Can you work these out from the model? Positions are in its coordinate system, mm. A direction names the side the tool comes from. Give positions to 0.01 mm unless a question says otherwise; leave off trailing zeros. Write each loop counter-clockwise with the first axis right and the second up, starting at its lowest first coordinate (ties: lowest second). Pieces come first, ordered by that corner, then holes.
1. On a 3-axis mill with a long thin cutter (end or side, diameter ignored), from which of +Z, -Z, +X, -X, +Y, -Y can I reach the whole of each face in a straight line? I mean faces 1 (the flat face through (4.5, 44, 1)), 2 (the flat face through (95.5, 44, 1)), 3 (the flat face through (130, 44, 1)). Say none if no direction works.
2. Suppose I cut it at D-D (y = 62). Please give me the cut outline in (x, z).
3. If I drill on probe 1 along Y at (x, z) = (101, 1.5); probe 2 along Y at (x, z) = (25, 2.05); probe 3 along Y at (x, z) = (72, 0.75), over which ranges is the centre line in solid material (lowest first)?
4. Suppose I cut it at C-C (z = 2.4). Please give me the cut outline in (x, y).
5. Suppose I cut it at A-A (x = 25). Please give me the cut outline in (y, z).
6. Thinking about a two-plate mould opening in Y: for faces 4 (the cylindrical face through (92.49, 66.15, 1.48)), 5 (the flat face through (0, 70, 1)), 6 (the cylindrical face through (4.28, 83.49, 1.48)), which applies, pulls with the +Y half, pulls with the -Y half, needs draft (parallel to the pull), parting line crosses it, or undercut?
7. I'm going to push a flat-ended pin straight in: pin 1 (0.9 mm diameter, centred on y = 51, z = 1.5, fed in from -X). Where does the tip first touch, or does it pass through?
8. Suppose I cut it at B-B (y = 40.5). Please give me the cut outline in (x, z), and give its area (4 significant figures).
Autodesk Inventor part; units mm, degrees
ref_plane "YZ Plane" through (0, 0, 0) normal (1, 0, 0) x (0, 1, 0)
ref_plane "XZ Plane" through (0, 0, 0) normal (0, 1, 0) x (-1, 0, 0)
ref_plane "XY Plane" through (0, 0, 0) normal (0, 0, 1) x (1, 0, 0)
sketch "Náčrt1" plane through (0, 0, 0) normal (0, 0, 1) x (1, 0, 0)
  line L0 (15, 0) -> (115, 0)
  line L1 (130, 15) -> (130, 73)
  line L2 (115, 88) -> (15, 88)
  line L3 (40.5, 69) -> (85.5, 69)
  line L4 (95.5, 59) -> (95.5, 29)
  line L5 (85.5, 19) -> (40.5, 19)
  line L6 (30.5, 29) -> (30.5, 59)
  arc A0 (40.5, 69) -> (30.5, 59) centre (40.5, 59) ccw
  arc A1 (95.5, 59) -> (85.5, 69) centre (85.5, 59) ccw
  arc A2 (85.5, 19) -> (95.5, 29) centre (85.5, 29) ccw
  arc A3 (30.5, 29) -> (40.5, 19) centre (40.5, 29) ccw
  arc A4 (130, 73) -> (115, 88) centre (115, 73) ccw
  arc A5 (115, 0) -> (130, 15) centre (115, 15) ccw
  arc A6 (15, 88) -> (0, 73) centre (15, 73) ccw
  arc A7 (0, 15) -> (15, 0) centre (15, 15) ccw
  circle A8 centre (25, 74) radius 2
  circle A9 centre (25, 14) radius 2
  circle A10 centre (101, 73) radius 2
  circle A11 centre (101, 15.1524) radius 2
  line L7 (4.5, 64) -> (4.5, 24)
  line L8 (4.5, 64) -> (0, 66.5981)
  line L9 (4.5, 24) -> (0, 21.4019)
  line L10 (0, 73) -> (0, 66.5981)
  line L11 (0, 21.4019) -> (0, 15)
  point P0 (0, 0)
  point P1 (30.5, 69)
  point P2 (95.5, 69)
  point P3 (30.5, 19)
  dimension "d0" = 65
  dimension "d1" = 50
  dimension "d7" = 34.5
  dimension "d9" = 88
  dimension "d10" = 19
  dimension "d16" = 76
  dimension "d18" = 60
  dimension "d19" = 14
  dimension "d23" = 105
  dimension "d24" = 0
extrude "Vysunutí1" add sketch "Náčrt1" along normal blind 3
properties part number "WarBRD_Upper_Plate"
Checks:
1. face 1: +Z, -Z, -X
1. face 2: +Z, -Z
1. face 3: +Z, -Z, +X, +Y, -Y
2. outline: (4.5, 0) - (30.96, 0) - (30.96, 3) - (4.5, 3) - close; (95.04, 0) - (130, 0) - (130, 3) - (95.04, 3) - close
3. probe 1: y = 0 to 13.15, 17.15 to 71, 75 to 88
3. probe 2: y = 0 to 12, 16 to 72, 76 to 88
3. probe 3: y = 0 to 19, 69 to 88
4. outline: (0, 15) arc R15 ccw to (15, 0) - (115, 0) arc R15 ccw to (130, 15) - (130, 73) arc R15 ccw to (115, 88) - (15, 88) arc R15 ccw to (0, 73) - (0, 66.6) - (4.5, 64) - (4.5, 24) - (0, 21.4) - close; hole circle Ø4 at (25, 14); hole circle Ø4 at (25, 74); hole (30.5, 29) arc R10 ccw to (40.5, 19) - (85.5, 19) arc R10 ccw to (95.5, 29) - (95.5, 59) arc R10 ccw to (85.5, 69) - (40.5, 69) arc R10 ccw to (30.5, 59) - close; hole circle Ø4 at (101, 15.15); hole circle Ø4 at (101, 73)
5. outline: (0, 0) - (12, 0) - (12, 3) - (0, 3) - close; (16, 0) - (72, 0) - (72, 3) - (16, 3) - close; (76, 0) - (88, 0) - (88, 3) - (76, 3) - close
6. face 4: undercut
6. face 5: needs draft
6. face 6: pulls with the +Y half
7. pin 1: stops at x = 4.5
8. outline: (4.5, 0) - (30.5, 0) - (30.5, 3) - (4.5, 3) - close; (95.5, 0) - (130, 0) - (130, 3) - (95.5, 3) - close
8. area: 181.5 mm2
